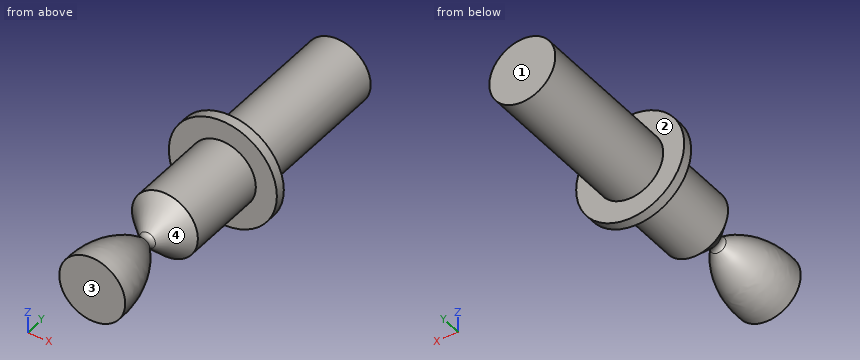
```python
from build123d import *

# Parameters (mm, degrees)
SKETCH2_W = 17
SKETCH2_H = 80


with BuildPart() as part:
    # Sketch1 → Revolve1 (revolve)
    with BuildSketch(Plane.XY):
        with BuildLine():
            Line((0, 0), (17, 0))
            ThreePointArc((17, 0), (14.146372017, 19.654148519), (4.091449674, 36.780948668))
            ThreePointArc((4.091449674, 36.780948668), (3.223460565, 38.876459746), (4.091449674, 40.971970825))
            Line((4.091449674, 40.971970825), (17, 53.880521151))
            Line((17, 53.880521151), (17, 96.852266261))
            Line((17, 96.852266261), (27.840575234, 96.852266261))
            Line((27.840575234, 96.852266261), (27.840575234, 102))
            Line((27.840575234, 102), (0, 102))
            Line((0, 102), (0, 0))
        make_face()
    revolve(axis=Axis((0, 0, 0), (0, 1, 0)))

    # Sketch2 → Revolve3 (revolve)
    with BuildSketch(Plane.XY):
        with Locations((8.5, 142)):
            Rectangle(SKETCH2_W, SKETCH2_H)
    revolve(axis=Axis((0, 102, 0), (0, 1, 0)))


solid = part.part
```
Input: part model. Units: mm. Frame: model coordinates. Face numbers are marked on the shaded views. A direction names the side the tool comes from. Round coordinates to 2 decimals unless told otherwise and drop trailing zeros. Loops run counter-clockwise (first coordinate to the right, second up) from the corner with the lowest first, then second, coordinate; pieces in that order, holes last. Notation, with made-up numbers: (16.25, 16) -> (57.25, 16) arc R28 cw to (57.25, 46) -> close; hole circle Ø5 at (-2.5, -34). An arc over 180 degrees is marked (long way). Write each question's results on one line, items separated by ' | '.
1. Ray query, line 1 (Y direction, x = -11, z = -24); line 2 (Y direction, x = 7, z = -3); line 3 (X direction, y = 96, z = -1). Return the intervals inside material, ascending. Write a range as from..to.
Geometry results:
line 1: 96.85..102 | line 2: 0..32.33, 44.5..182 | line 3: -16.97..16.97
2. Set-up query: the marked faces 1 and 2. Return all of +Z, -Z, +X, -X, +Y, -Y with unobstructed straight access to the full face (end or side cutting, diameter ignored); none if empty.
Geometry results:
face 1: +Z, -Z, +X, -X, +Y | face 2: +Y
3. Section A-A (y = 87). Return loops of the section in (x, z), and give its area (3 significant figures).
Geometry results:
outline: circle Ø34 at (0, 0) | area: 908 mm2
4. Mould query, pull axis Y, two halves, no side actions, for the marked faces 3 and 4. Classes: +Y half, -Y half, draft (parallel to the pull), parting line (faces both ways), or undercut.
Geometry results:
face 3: -Y half | face 4: undercut
5. First-contact query: P1, Ø2, axis at x = -10, y = 26.5, coming from the +Z side; P2, Ø6, axis at x = 1, y = 75, coming from the +Z side; P3, Ø2, axis at x = -9.5, y = 73.5, coming from the +Z side; P4, Ø1.5, axis at y = 130.5, z = 19, coming from the -X side. Flat tips, straight axial feed; report the tip coordinate or a pass-through.
Geometry results:
P1: z = 6.87 | P2: z = 17 | P3: z = 14.72 | P4: through
